For this review, take the finished solid that the model builds, in its own axes (mm). A direction names the side the tool comes from. Give positions to 0.01 mm unless a question says otherwise; leave off trailing zeros. Write each loop counter-clockwise with the first axis right and the second up, starting at its lowest first coordinate (ties: lowest second). Pieces come first, ordered by that corner, then holes. Notation, with made-up numbers: M -1.5,87.25 L 23.5,87.25 A20 cw 23.5,104.25 Z; hole C -6.5,64.25 d11. An arc over 180 degrees is marked long. Use one line per item in the form item = value. Start each with the question number.
Q1. Consider section C-C on z = 706. Write out the cut boundary in (x, y), and give its area (3 significant figures).
Q2. Consider section A-A on x = -11. Write out the cut boundary in (y, z), and give its area (3 significant figures).
Q3. Tool access review of faces 1 (the flat face through (0, 15, 410)), 2 (the flat face through (21.1, 95, 15)), 3 (the flat face through (21.1, 0, 410)): name each direction out of +Z, -Z, +X, -X, +Y, -Y from which nothing blocks a thin tool from reaching the whole face with its end or side.
Q4. Consider section B-B on y = 148.5. Write out the cut boundary in (x, z), and give its area (3 significant figures).
Q5. Clearance check with flat-ended pins moving along their axes: pin 1 Ø9 at (y, z) = (1, 357) entering from +X; pin 2 Ø24 at (x, z) = (67.5, 16.5) entering from +Y. State where each tip first meets the part, or that it passes through.
Q6. For probe 1 along Z at (x, y) = (1, 65); probe 2 along X at (y, z) = (5, 616.5); probe 3 along Y at (x, z) = (-3.5, 232.5), list the stretches that pass through material, from the lowest coordinate up. Write a range as [from, to].
```python
from build123d import *

# Parameters (mm, degrees)
F0_W     = 42.2
F0_H     = 30
F1_DEPTH = 800
F2_DEPTH = 30


with BuildPart() as f1:
    # F0 (on Top) → F1 (new body)
    with BuildSketch(Plane.XY):
        Rectangle(F0_W, F0_H)
    extrude(amount=F1_DEPTH)

    # F0 (on Top) → F2 (join)
    with BuildSketch(Plane.XY):
        Polygon((21.1, 15), (21.1, -15), (111.1, -15), (111.1, 27.2), (21.1, 27.2), align=None)
        Polygon((-21.1, 15), (21.1, 15), (21.1, 27.2), (21.1, 165), (-21.1, 165), align=None)
    extrude(amount=F2_DEPTH)


solid = f1.part
```
Working result:
q1.outline = M -21.1,-15 L 21.1,-15 L 21.1,15 L -21.1,15 Z
q1.area = 1,270 mm²
q2.outline = M -15,0 L 165,0 L 165,30 L 15,30 L 15,800 L -15,800 Z
q2.area = 28,500 mm²
q3.face_1 = +Z, +X, -X, +Y
q3.face_2 = +Z, -Z, +X, +Y
q3.face_3 = +Z, +X, +Y, -Y
q4.outline = M -21.1,0 L 21.1,0 L 21.1,30 L -21.1,30 Z
q4.area = 1,270 mm²
q5.pin_1 = 21.1
q5.pin_2 = 27.2
q6.probe_1 = [0, 30]
q6.probe_2 = [-21.1, 21.1]
q6.probe_3 = [-15, 15]
